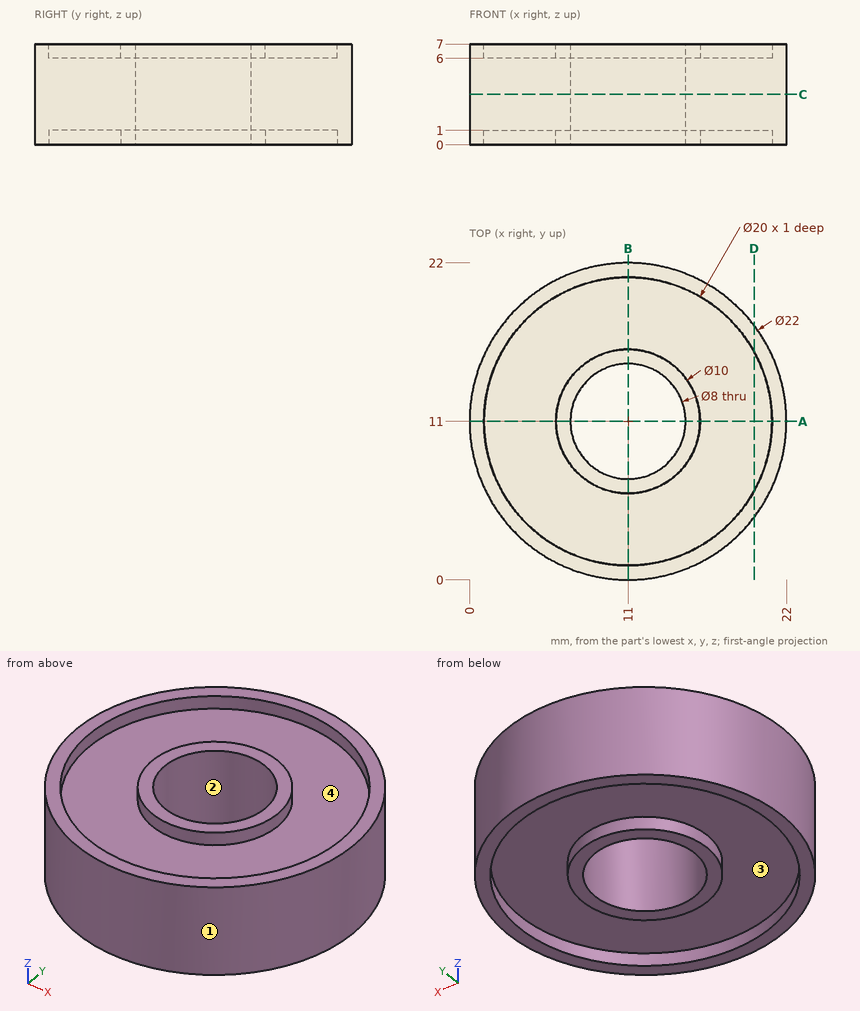
The figure shows three views and two pictorial views of one solid part (mm, origin at its lowest corner). Answer the questions. A direction names the side the tool comes from. Round coordinates to 2 decimals unless told otherwise and drop trailing zeros. Write each loop counter-clockwise with the first axis right and the second up, starting at its lowest first coordinate (ties: lowest second). Pieces come first, ordered by that corner, then holes. Notation, with made-up numbers: (-8.5, 45.25) -> (24.5, 45.25) arc R12 cw to (24.5, 62.25) -> close; hole circle Ø1 at (12.25, 43.5). An arc over 180 degrees is marked (long way). Answer as a JSON object with one key per item and string values. Group by question number.
Q1. Section D-D (x = 19.75) is taken. Write down the section's boundary in (y, z), plus the area to 3 significant figures.
Q2. Straight lines are drawn through the part: line 1 along Y through (x, z) = (11, 0.7); line 2 along Y through (x, z) = (11, 4.5); line 3 along Y through (x, z) = (11.75, 6.75). For each, find the intervals that lie inside material, in ascending order.
Q3. Section C-C (z = 3.5) is taken. Write down the section's boundary in (x, y).
Q4. Which of the six approach directions +Z, -Z, +X, -X, +Y, -Y give full straight-line access (tool end or side, diameter ignored) to the marked faces 3 and 4?
Q5. Section A-A (y = 11) is taken. Write down the section's boundary in (x, z).
Q6. Each of these flat-tipped pins is pushed along its axis until it touches: pin 1 Ø13 at (x, y) = (11, 11) entering from -Z; pin 2 Ø3 at (x, z) = (14.5, 1) entering from +Y; pin 3 Ø2 at (x, z) = (7, 4) entering from +Y; pin 4 Ø4 at (y, z) = (16, 2) entering from +X. Where does it stop, or does it pass through?
Q7. Determine the mould class of the marked faces 1 and 2 for opening direction X: pulls with the +X half, pulls with the -X half, needs draft (parallel to the pull), parting line crosses it, or undercut.
Check values:
{
 "1": {"outline": "(4.33, 0) -> (6.16, 0) -> (6.16, 1) -> (15.84, 1) -> (15.84, 0) -> (17.67, 0) -> (17.67, 7) -> (15.84, 7) -> (15.84, 6) -> (6.16, 6) -> (6.16, 7) -> (4.33, 7) -> close", "area": "74.0 mm^2"},
 "2": {"line 1": "0 to 1, 6 to 7, 15 to 16, 21 to 22", "line 2": "0 to 7, 15 to 22", "line 3": "0.03 to 1.03, 6.06 to 7.07, 14.93 to 15.94, 20.97 to 21.97"},
 "3": {"outline": "circle Ø22 at (11, 11); hole circle Ø8 at (11, 11)"},
 "4": {"face 3": "-Z", "face 4": "+Z"},
 "5": {"outline": "(0, 0) -> (1, 0) -> (1, 1) -> (6, 1) -> (6, 0) -> (7, 0) -> (7, 7) -> (6, 7) -> (6, 6) -> (1, 6) -> (1, 7) -> (0, 7) -> close; (15, 0) -> (16, 0) -> (16, 1) -> (21, 1) -> (21, 0) -> (22, 0) -> (22, 7) -> (21, 7) -> (21, 6) -> (16, 6) -> (16, 7) -> (15, 7) -> close"},
 "6": {"pin 1": "z = 0", "pin 2": "y = 21.82", "pin 3": "y = 21.58", "pin 4": "x = 21.58"},
 "7": {"face 1": "parting line crosses it", "face 2": "undercut"}
}
